```python
from build123d import *

# Parameters (mm, degrees)
CROQUIS1_R              = 29
SALIENTE_EXTRUIR1_DEPTH = 5
CROQUIS2_R              = 24
CROQUIS3_R              = 39
CROQUIS4_R              = 65
SALIENTE_EXTRUIR2_DEPTH = 5
SALIENTE_EXTRUIR3_START = 5
CROQUIS5_R              = 65
CROQUIS5_R_2            = 62.5
SALIENTE_EXTRUIR3_DEPTH = 5
REDONDEO1_R             = 5
CROQUIS6_R              = 23
CORTAR_EXTRUIR1_DEPTH   = 62
REDONDEO2_R             = 3


with BuildPart() as part:
    # Croquis1 → Saliente-Extruir1 (new body)
    with BuildSketch(Plane(origin=(0, 0, 0), x_dir=(1, 0, 0), z_dir=(0, 1, 0))):
        with Locations(Location((0, 0, 0), (0, 0, 270))):
            Circle(CROQUIS1_R)
    extrude(amount=SALIENTE_EXTRUIR1_DEPTH)

    # Croquis2 → Recubrir1 section 0
    with BuildSketch(Plane(origin=(0, 5, 0), x_dir=(1, 0, 0), z_dir=(0, 1, 0))):
        Circle(CROQUIS2_R)
    # Croquis3 → Recubrir1 section 1
    with BuildSketch(Plane(origin=(0, 135, 0), x_dir=(1, 0, 0), z_dir=(0, 1, 0))):
        Circle(CROQUIS3_R)
    loft()

    # Croquis4 → Saliente-Extruir2 (add)
    with BuildSketch(Plane(origin=(0, 135, 0), x_dir=(1, 0, 0), z_dir=(0, 1, 0))):
        with Locations(Location((0, 0, 0), (0, 0, 270))):
            Circle(CROQUIS4_R)
    extrude(amount=SALIENTE_EXTRUIR2_DEPTH)

    # Croquis5 → Saliente-Extruir3 (add)
    with BuildSketch(Plane.XZ.offset(-135).offset(SALIENTE_EXTRUIR3_START)):
        with Locations(Location((0, 0, 0), (0, 0, 270))):
            Circle(CROQUIS5_R)
        with Locations(Location((0, 0, 0), (0, 0, 270))):
            Circle(CROQUIS5_R_2, mode=Mode.SUBTRACT)
    extrude(amount=-SALIENTE_EXTRUIR3_DEPTH)

    # Redondeo1
    redondeo1_edges = [part.edges().sort_by_distance(p)[0] for p in [
        (0, 140, -65),
        (0, 135, 62.5),
        (0, 5, -29),
    ]]
    fillet(redondeo1_edges, radius=REDONDEO1_R - 0.0001)  # a hair under: the kernel refuses the full size

    # Croquis6 → Cortar-Extruir1 (cut)
    with BuildSketch(Plane.XZ):
        with Locations(Location((0, 0, 0), (0, 0, 270))):
            Circle(CROQUIS6_R)
    extrude(amount=-CORTAR_EXTRUIR1_DEPTH, mode=Mode.SUBTRACT)

    # Croquis7 → Cortar-Revolución1 (revolve, cut)
    with BuildSketch(Plane.XY, mode=Mode.PRIVATE) as cortar_revoluci_n1_sk:
        Polygon((22, 37.952055194), (0, 37.952055194), (0, 140), (34, 140), align=None)
    revolve(cortar_revoluci_n1_sk.sketch.rotate(Axis((0, 192.821641375, 0), (0, -1, 0)), 90), axis=Axis((0, 192.821641375, 0), (0, -1, 0)), mode=Mode.SUBTRACT)

    # Redondeo2
    redondeo2_edges = [part.edges().sort_by_distance(p)[0] for p in [
        (-24, 5, 0),
    ]]
    fillet(redondeo2_edges, radius=REDONDEO2_R)


solid = part.part
```
Source: CAD feature listing. Evaluate the final solid. Frame: model axes, mm. A direction names the side the tool comes from. Give positions to 0.01 mm unless a question says otherwise; leave off trailing zeros. Loops run counter-clockwise (first coordinate to the right, second up) from the corner with the lowest first, then second, coordinate; pieces in that order, holes last. Notation, with made-up numbers: (28.5, -20) -> (71.5, -20) arc R19 ccw to (71.5, 4) -> close; hole circle Ø9 at (29.25, 48.5). An arc over 180 degrees is marked (long way). Use a Markdown table: item, result. Add a question column.
(1) Access query for faces 3 (the face through (29.334, 72.211, 12.162)), 4 (the face through (53, 130, 34)), 5 (the face through (-26, 140, 26)). Directions: +Z, -Z, +X, -X, +Y, -Y. A direction counts if a zero-diameter tool reaches every point of the face in a straight line with its end or side. Return the directions, or none.
(2) First-contact query: pin 1 Ø1 at (y, z) = (117, -13.5) entering from +X; pin 2 Ø6 at (y, z) = (105, 29.5) entering from -X; pin 3 Ø10 at (x, y) = (3.5, 26) entering from +Z. Flat tips, straight axial feed; report the tip coordinate or a pass-through.
(3) Pull-direction query (X, two-part tool) for faces 1 (the face through (-8.54, 92.57, 27.11)), 2 (the face through (22, 0, -9)); classes: +X half, -X half, draft (parallel to the pull), parting line (faces both ways), or undercut.
(4) Ray query, line 1 (X direction, y = 130.05, z = 0); line 2 (Y direction, x = -27.5, z = -33.5); line 3 (X direction, y = 27.5, z = 0). Return the intervals inside material, ascending.
(5) Section query B-B (y = 12). Output: boundary loops of the cut face in (x, z).
(6) Section query A-A (y = 26). Output: boundary loops of the cut face in (x, z), then the cut area to 3 significant figures.
Checked values:
| question | item | result |
|---|---|---|
| 1 | face 3 | none |
| 1 | face 4 | -Y |
| 1 | face 5 | +Z, -Z, +X, -X, +Y |
| 2 | pin 1 | x = 34.57 |
| 2 | pin 2 | x = -23.72 |
| 2 | pin 3 | z = 26.91 |
| 3 | face 1 | undercut |
| 3 | face 2 | draft |
| 4 | line 1 | -65 to -62.5, -38.43 to -32.83, 32.83 to 38.43, 62.5 to 65 |
| 4 | line 2 | 135 to 140 |
| 4 | line 3 | -26.6 to -23, 23 to 26.6 |
| 5 | outline | circle Ø49.62 at (0, 0); hole circle Ø46 at (0, 0) |
| 6 | outline | circle Ø52.85 at (0, 0); hole circle Ø46 at (0, 0) |
| 6 | area | 531 mm^2 |
